```python
from build123d import *

# Parameters (mm, degrees)
F0_R     = 40
F1_DEPTH = 15
F0_R_2   = 25
F2_DEPTH = 150
F3_DEPTH = 30
F4_DEPTH = 8


# Not quite as in the source:
# - ends of sketch curves that miss each other by under 0.0002 mm in the source are joined


with BuildPart() as f1:
    # F0 (on Front) → F1 (new body)
    with BuildSketch(Plane.XZ):
        with BuildLine():
            ThreePointArc((136.9199448282, 386.2104516544), (124.4705090254, 391.3857217921), (111.4380638613, 394.8393062852))
            Line((111.4380638613, 394.8393062852), (42.918713, 408.129393))
            ThreePointArc((42.918713, 408.129393), (-22.539049679, 352.8547276711), (45.4216669824, 300.6881840726))
            Line((45.4216669824, 300.6881840726), (102.160582, 314.462893))
            ThreePointArc((102.160582, 314.462893), (116.5305641711, 315.8079808018), (130.6860790256, 312.992479072))
            ThreePointArc((130.6860790256, 312.992479072), (204.0553442227, 304.6657026983), (273.5865736459, 329.5211325506))
            ThreePointArc((273.5865736459, 329.5211325506), (289.1363732598, 337.5026610827), (306.4832439925, 339.6444218586))
            Line((306.4832439925, 339.6444218586), (530.552186, 327.792845))
            ThreePointArc((530.552186, 327.792845), (559.0680406559, 322.0478617496), (584.7240709532, 308.3392179368))
            ThreePointArc((584.7240709532, 308.3392179368), (672.2592374085, 348.3136045992), (591.9275499624, 401.2964030718))
            ThreePointArc((591.9275499624, 401.2964030718), (564.8093719906, 391.7707004398), (536.1018479581, 390.3520205594))
            Line((536.1018479581, 390.3520205594), (279.382043, 414.771009))
            ThreePointArc((279.382043, 414.771009), (255.4725507994, 411.172762836), (236.0470033399, 396.7762595435))
            ThreePointArc((236.0470033399, 396.7762595435), (188.0244125036, 377.0364695299), (136.9199448282, 386.2104516544))
        make_face()
        with Locations((32.446032, 354.135662)):
            Circle(F0_R, mode=Mode.SUBTRACT)
        with Locations((617.423637, 352.562949)):
            Circle(F0_R, mode=Mode.SUBTRACT)
    extrude(amount=F1_DEPTH)

    # F0 (on Front) → F2 (join)
    with BuildSketch(Plane.XZ):
        with Locations((32.446032, 354.135662)):
            Circle(F0_R)
        with Locations((32.446032, 354.135662)):
            Circle(F0_R_2, mode=Mode.SUBTRACT)
    extrude(amount=F2_DEPTH)

    # F0 (on Front) → F3 (join)
    with BuildSketch(Plane.XZ):
        with Locations((617.423637, 352.562949)):
            Circle(F0_R)
        with Locations((617.423637, 352.562949)):
            Circle(F0_R_2, mode=Mode.SUBTRACT)
    extrude(amount=F3_DEPTH)

    # F0 (on Front) → F4 (join)
    with BuildSketch(Plane.XZ):
        with Locations((617.423637, 352.562949)):
            Circle(F0_R)
        with Locations((617.423637, 352.562949)):
            Circle(F0_R_2, mode=Mode.SUBTRACT)
    extrude(amount=-F4_DEPTH)


solid = f1.part
```
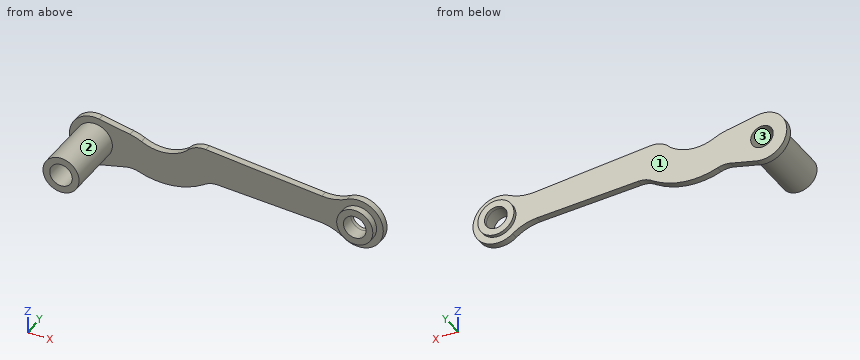
Read the model definition and answer for the solid it produces. Units are mm, in the model's axes. Face numbers are marked on the shaded views. Give positions to 0.01 mm unless a question says otherwise; leave off trailing zeros. Order: outer loops, then holes, each group sorted by start corner. A loop starts at its lowest first (then second) coordinate and runs counter-clockwise, first axis right, second up.
(1) Find section A-A (z = 364). Give the vertices of the cut face in (x, y).
(2) Find section D-D (x = 87). Give the vertices of the cut face in (y, z).
(3) Find section C-C (y = -57). Give the vertices of the cut face in (x, z).
(4) Find section B-B (x = 600.5). Give the vertices of the cut face in (y, z), plus the area to 3 significant figures.
(5) For a pull along Z with two mould halves and no side action, classify the marked faces 1, 2 and 3 as released by +Z, released by -Z, zero draft, split by the parting line, or undercut.
(6) Given pin 1 (2 mm diameter, centred on x = 286.5, z = 364.5, fed in from -Y); pin 2 (3 mm diameter, centred on x = 471, z = 375.5, fed in from +Y); pin 3 (1.5 mm diameter, centred on y = -35, z = 341, fed in from +X), each flat-ended and moving along its own axis, determine where each tip first touches the part or whether it passes through.
(7) Straight lines are drawn through the part: L1, parallel to Z at x = 620, y = -17.5; L2, parallel to Y at x = 617.5, z = 400.5; L3, parallel to X at y = -17, z = 370. For each, find the intervals that lie inside material, in ascending order.
Result sheet:
1. outline: (-21.66, -15) - (-6.32, -15) - (-6.32, -150) - (9.47, -150) - (9.47, 0) - (-21.66, 0) - close; (55.42, -150) - (71.21, -150) - (71.21, -15) - (579.09, -15) - (579.09, -30) - (595.19, -30) - (595.19, 8) - (579.09, 8) - (579.09, 0) - (55.42, 0) - close; (639.65, -30) - (655.75, -30) - (655.75, -15) - (671.22, -15) - (671.22, 0) - (655.75, 0) - (655.75, 8) - (639.65, 8) - close
2. outline: (-15, 310.78) - (0, 310.78) - (0, 399.58) - (-15, 399.58) - close
3. outline: circle Ø80 at (32.45, 354.14); hole circle Ø50 at (32.45, 354.14)
4. outline: (-30, 316.32) - (-15, 316.32) - (-15, 300.23) - (0, 300.23) - (0, 316.32) - (8, 316.32) - (8, 334.16) - (-30, 334.16) - close; (-30, 370.96) - (8, 370.96) - (8, 388.81) - (0, 388.81) - (0, 404.89) - (-15, 404.89) - (-15, 388.81) - (-30, 388.81) - close
4. area: 1,840 mm2
5. face 1: zero draft
5. face 2: split by the parting line
5. face 3: undercut
6. pin 1: stops at y = -15
6. pin 2: stops at y = 0
6. pin 3: stops at x = 70.48
7. L1: z = 312.65 to 327.7, 377.43 to 392.48
7. L2: y = -15 to 0
7. L3: x = -4.27 to 13.12, 51.77 to 69.17, 581.42 to 599.51, 635.34 to 653.42
